from build123d import *

# Parameters (mm, degrees)
M8_GEWINDEBOHRUNG1_D     = 6.8
M8_GEWINDEBOHRUNG1_DEPTH = 15
M8_GEWINDEBOHRUNG1_TIP   = 2.042926105
FASE1_SIZE               = 1
FASE2_SIZE               = 1


with BuildPart() as part:
    # Skizze1 → Rotation1 (revolve)
    with BuildSketch(Plane.XY):
        Polygon((0, 0), (-8, 0), (-8, 32), (-6, 32), (-6, 52), (0, 52), align=None)
    revolve(axis=Axis((0, 66.923871734, 0), (0, -1, 0)))

    # M8 Gewindebohrung1
    with Locations(Plane(origin=(0, 0, 0), x_dir=(-1, 0, 0), z_dir=(0, -1, 0))):
        with Locations((0, 0)):
            Hole(M8_GEWINDEBOHRUNG1_D / 2, depth=M8_GEWINDEBOHRUNG1_DEPTH)
            with Locations((0, 0, -(M8_GEWINDEBOHRUNG1_DEPTH + M8_GEWINDEBOHRUNG1_TIP / 2))):  # 118° drill point
                Cone(0, M8_GEWINDEBOHRUNG1_D / 2, M8_GEWINDEBOHRUNG1_TIP, mode=Mode.SUBTRACT)

    # Fase1
    fase1_edges = [part.edges().sort_by_distance(p)[0] for p in [
        (6, 52, 0),
    ]]
    chamfer(fase1_edges, length=FASE1_SIZE)

    # Fase2
    fase2_edges = [part.edges().sort_by_distance(p)[0] for p in [
        (8, 32, 0),
    ]]
    chamfer(fase2_edges, length=FASE2_SIZE)


solid = part.part
The model under review builds one solid part; all positions refer to its coordinate system, in mm. A direction names the side the tool comes from. Round coordinates to 2 decimals unless told otherwise and drop trailing zeros. Loops run counter-clockwise (first coordinate to the right, second up) from the corner with the lowest first, then second, coordinate; pieces in that order, holes last. Notation, with made-up numbers: (46, -1) -> (83, -1) arc R15 cw to (83, 7) -> close; hole circle Ø1 at (-8.75, 19). An arc over 180 degrees is marked (long way). Write item = value, one per line. Start each with the question number.
Item 1: Take a section at A-A on y = 9. Give the boundary of the cut face in (x, z), plus the area to 3 significant figures.
Item 2: Take a section at B-B on y = 36. Give the boundary of the cut face in (x, z), plus the area to 3 significant figures.
Item 3: For faces 4 (the cylindrical face through (1.73, 15.72, 7.81)), 5 (the flat face through (-6, 32, -2)), list the 3-axis set-ups (+Z, -Z, +X, -X, +Y, -Y) from which the entire face can be reached by the end or side of a thin tool; tool diameter is ignored.
Item 4: Mouldability with a two-part tool opening along Z and no side actions: class faces 1 (the flat face through (3, 0, 2)), 2 (the cylindrical face through (-0.74, 7.6, 3.32)), 3 (the cylindrical face through (6, 42, 0)) as released by +Z, released by -Z, zero draft, split by the parting line, or undercut.
Item 5: Insertion check: pin 1 (6 mm diameter, centred on x = -1.5, y = 38.5, fed in from +Z); pin 2 (1 mm diameter, centred on y = 19, z = -6, fed in from +X); pin 3 (1.5 mm diameter, centred on y = 41.5, z = 4, fed in from +X). Each pin has a flat end and moves straight along its axis. Give the tip position at first contact, or say it passes through.
Item 6: To check wall thickness, follow L1, parallel to Z at x = 0, y = 4.25; L2, parallel to X at y = 13.5, z = -0.25; L3, parallel to Y at x = 2.25, z = -6.25. State the ranges of each line that lie inside material, in increasing order.
Result:
q1.outline = circle Ø16 at (0, 0); hole circle Ø6.8 at (0, 0)
q1.area = 165 mm²
q2.outline = circle Ø12 at (0, 0)
q2.area = 113 mm²
q3.face_4 = +Y, -Y
q3.face_5 = +Y
q4.face_1 = zero draft
q4.face_2 = undercut
q4.face_3 = split by the parting line
q5.pin_1 = 6
q5.pin_2 = 5.81
q5.pin_3 = 5.04
q6.L1 = -8 to -3.4, 3.4 to 8
q6.L2 = -8 to -3.39, 3.39 to 8
q6.L3 = 0 to 32
